Geometry: see drawing. Coordinates: mm, zero at the bounding-box minimum. Coordinates: 2 decimals unless noted, no trailing zeros. Loops run counter-clockwise (first coordinate to the right, second up) from the corner with the lowest first, then second, coordinate; pieces in that order, holes last.
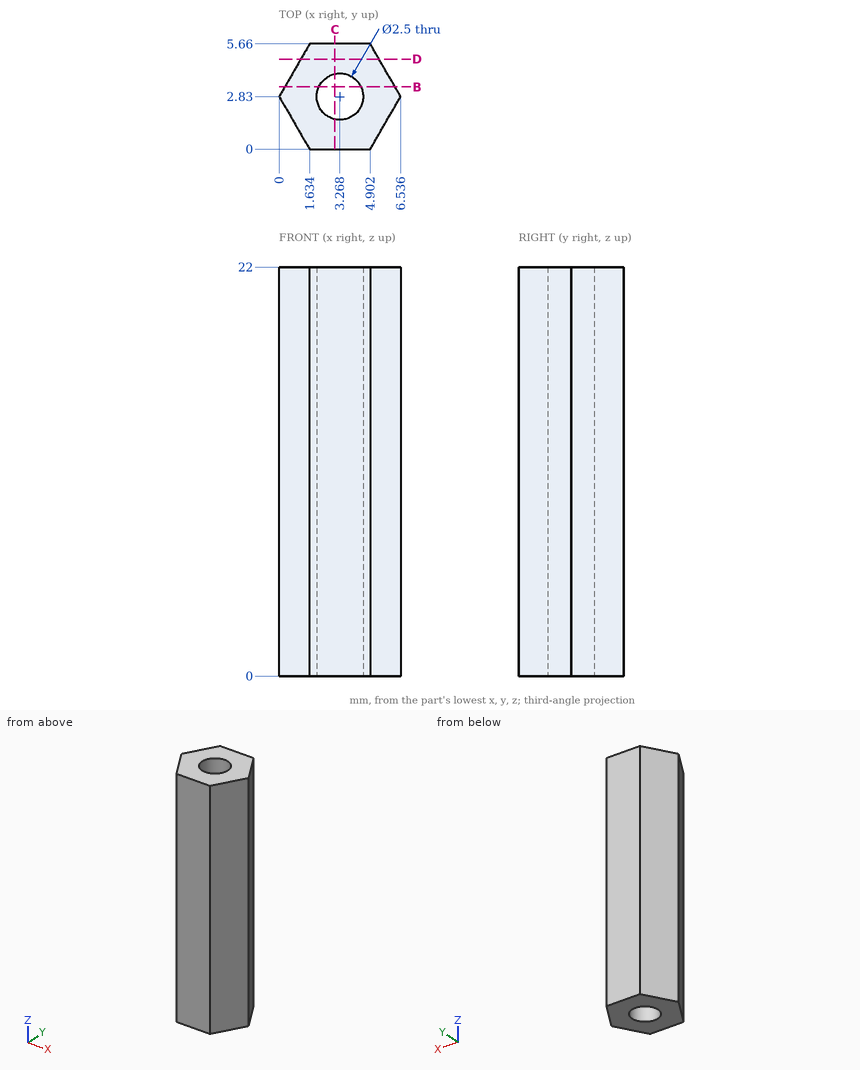
Item 1: Line query: L1, parallel to X at y = 2.5, z = 10.5 (1 decimal); L2, parallel to Y at x = 2.5, z = 12.5 (1 decimal); L3, parallel to X at y = 2.25, z = 12.25 (1 decimal). Output: solid intervals per line, ascending.
Result:
L1: x = 0.2 to 2.1, 4.5 to 6.3
L2: y = 0 to 1.8, 3.8 to 5.7
L3: x = 0.3 to 2.2, 4.4 to 6.2
Item 2: Section query B-B (y = 3.35). Output: boundary loops of the cut face in (x, z) (1 decimal).
Result:
outline: (0.3, 0) - (2.1, 0) - (2.1, 22) - (0.3, 22) - close; (4.4, 0) - (6.2, 0) - (6.2, 22) - (4.4, 22) - close
Item 3: Section query D-D (y = 4.85). Output: boundary loops of the cut face in (x, z).
Result:
outline: (1.17, 0) - (5.37, 0) - (5.37, 22) - (1.17, 22) - close
Item 4: Section query C-C (x = 3). Output: boundary loops of the cut face in (y, z).
Result:
outline: (0, 0) - (1.61, 0) - (1.61, 22) - (0, 22) - close; (4.05, 0) - (5.66, 0) - (5.66, 22) - (4.05, 22) - close
Item 5: Contact query for flat-ended pins moving along their axis: P1, Ø2, axis at x = 2.5, y = 1.5, coming from the -Z side; P2, Ø1, axis at y = 5, z = 3, coming from the +X side; P3, Ø2, axis at y = 5, z = 12.5, coming from the +X side. Output: stop coordinate, or through.
Result:
P1: stops at z = 0
P2: stops at x = 5.57
P3: stops at x = 5.86
